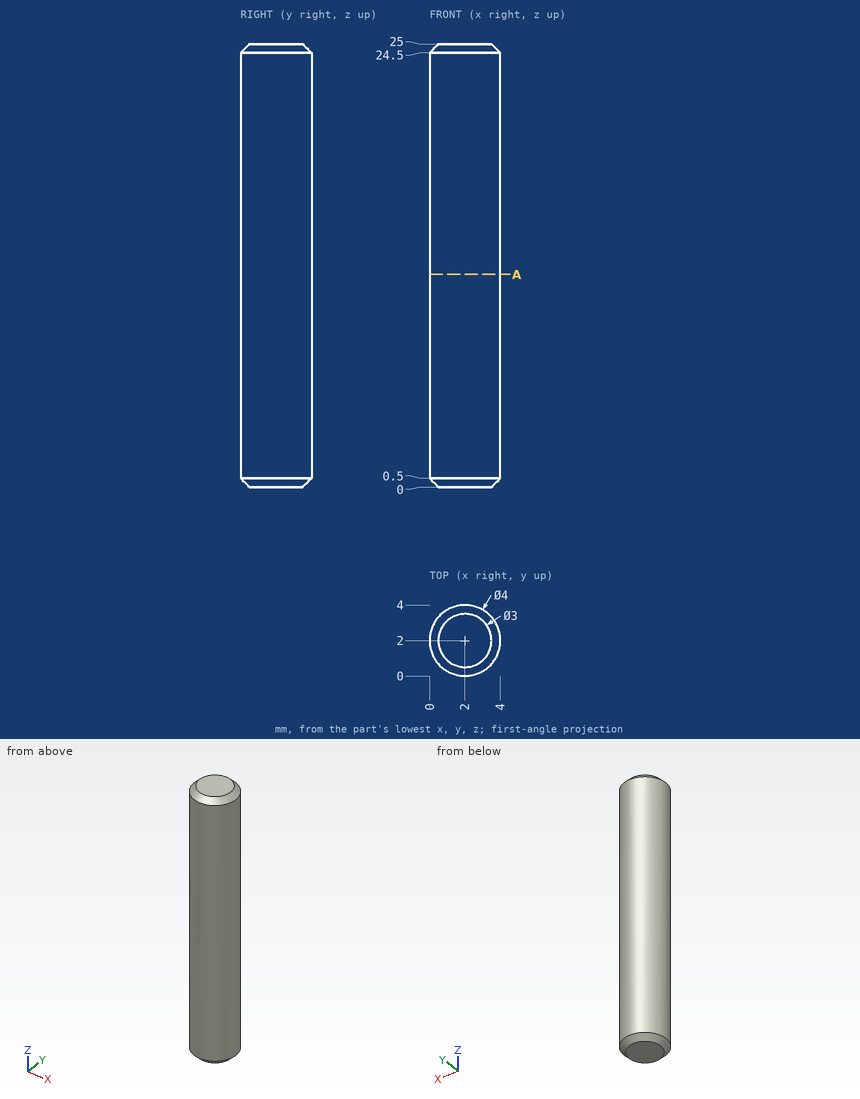
The figure shows three views and two pictorial views of one solid part (mm, origin at its lowest corner). Answer the questions. Give positions to 0.01 mm unless a question says otherwise; leave off trailing zeros. Order: outer loops, then holes, each group sorted by start corner. A loop starts at its lowest first (then second) coordinate and runs counter-clockwise, first axis right, second up. Notation, with made-up numbers: (-14.75, 56.25) -> (4.25, 56.25) arc R29 cw to (4.25, 76.25) -> close; hole circle Ø7 at (37, -3.5). An arc over 180 degrees is marked (long way). Answer as CSV lines item,"result". Start each with the question number.
(1) Each of these flat-tipped pins is pushed along its axis until it touches: pin 1 Ø1 at (x, z) = (3.5, 18.5) entering from +Y; pin 2 Ø1.5 at (x, z) = (3, 10) entering from -Y. Where does it stop, or does it pass through?
(2) Section A-A, the plane z = 12 is taken. Write down the section's boundary in (x, y), plus the area to 3 significant figures.
(3) Consider line 1 along X through (y, z) = (1.9, 7.5); line 2 along Y through (x, z) = (1.4, 17.75); line 3 along X through (y, z) = (1, 17.5). Determine where each line is inside the solid, lowest interval first.
Entries:
1,pin 1,"y = 3.73"
1,pin 2,"y = 0.02"
2,outline,"circle Ø4 at (2, 2)"
2,area,"12.6 mm²"
3,line 1,"0 to 4"
3,line 2,"0.09 to 3.91"
3,line 3,"0.27 to 3.73"
